Verification items for the finished model (mm, model axes). A direction names the side the tool comes from. Coordinates: 2 decimals unless noted, no trailing zeros. Order: outer loops, then holes, each group sorted by start corner. A loop starts at its lowest first (then second) coordinate and runs counter-clockwise, first axis right, second up. Notation, with made-up numbers: (19, -29) -> (77, -29) arc R26 ccw to (77, -7) -> close; hole circle Ø2 at (66, 65.5). An arc over 180 degrees is marked (long way). Write item = value, one per line. Start each with the question number.
1. Thickness scan on line 1 along Z through (x, y) = (76.9, 8.5); line 2 along X through (y, z) = (4.5, -28); line 3 along X through (y, z) = (2, 5). Record the ranges inside material, lowest first. Write a range as from..to.
2. Cross-section at A-A on y = 4.75. Record the cut outline in (x, z), plus the area to 3 significant figures.
3. Release check for a two-part mould opening along Z. For faces 4 (the flat face through (9, 2, -5)), 5 (the conical face through (77.115, 2.379, -28.028)), 6 (the flat face through (12, 10, -27)) record: +Z half, -Z half, draft (parallel to the pull), parting line (faces both ways), or undercut.
4. Cross-section at C-C on x = 57.5. Record the cut outline in (y, z).
5. Go/stop test with flat-tipped pins: P1, Ø5, axis at x = 60, y = 1.5, coming from the +Z side; P2, Ø2, axis at y = 1, z = 4.5, coming from the +X side; P3, Ø2, axis at x = 11, z = 18, coming from the -Y side; P4, Ø4.5, axis at y = 1.5, z = -20.5, coming from the -X side. Record where each tip stops, or that it passes through.
6. Cross-section at B-B on z = 3.5. Record the cut outline in (x, y).
7. Set-up check for faces 1 (the flat face through (78, 10, 19)), 2 (the cylindrical face through (75.846, 6.451, -27.328)), 3 (the flat face through (13, 2, 6)): record each of +Z, -Z, +X, -X, +Y, -Y from which the full face is reachable in a straight line by a thin tool's end or side.
Autodesk Fusion 360 part; units mm, degrees
sketch "Schizzo9" plane through (0, 0, 0) normal (0, 1, 0) x (1, 0, 0)
  line L0 (11, 28) -> (76.9, 28)
  line L1 (76.9, 28) -> (76.9, -18)
  line L2 (76.9, -18) -> (11, -18)
  line L3 (11, -18) -> (11, 28)
  circle A0 centre (11, 28) radius 2.75
  circle A1 centre (76.9, 28) radius 2.75
  circle A2 centre (11, -18) radius 2.75
  circle A3 centre (76.9, -18) radius 2.75
  line L4 (11, 28) -> (9, 28)
  line L5 (11, 28) -> (13, 28)
  line L6 (9, 28) -> (9, -18)
  line L7 (13, 28) -> (13, -18)
  line L8 (76.9, 28) -> (74.9, 28)
  line L9 (76.9, 28) -> (78.9, 28)
  line L10 (78.9, 28) -> (78.9, -18)
  line L11 (74.9, 28) -> (74.9, -18)
  line L12 (78.9, 5) -> (78.9, 7)
  line L13 (78.9, 5) -> (78.9, 3)
  line L14 (78.9, 7) -> (9, 7)
  line L15 (78.9, 3) -> (9, 3)
  dimension "d99" = 65.9
  dimension "d100" = 46
  dimension "d101" = 5.5
  dimension "d102" = 5.5
  dimension "d103" = 5.5
  dimension "d104" = 5.5
  dimension "d105" = 2
  dimension "d106" = 2
  dimension "d107" = 2
  dimension "d108" = 2
  dimension "d109" = 2
  dimension "d110" = 2
extrude "Estrusione16" add sketch "Schizzo9" along normal blind 4 contours L3 A0 L7 L14 | L3 A0 L6 L14 | L3 L7 L14 L15 | L3 L6 L14 L15 | L7 L11 L14 L15 | L3 A2 L7 L15 | L3 A2 L6 L15 | L1 A1 L11 L14 | L1 L11 L14 L15 | L1 A1 L10 L14 | L1 A3 L11 L15 | L1 L10 L12 L13 L14 L15 | L1 A3 L10 L15
extrude "Estrusione17" add sketch "Schizzo9" along normal blind 10 contours L0 A0 L4 L5 L6 | L0 L3 A0 L5 L7 | L3 A0 L4 L6 | L0 A0 L7 | L0 A1 L8 L9 L10 | L0 A1 L11 | L0 L1 A1 L8 L11 | L2 L3 A2 L7 | L2 L3 A2 | L1 A1 L9 L10 | L2 A2 L7 | L2 A3 L11 | L1 L2 A3 L11 | L1 L2 A3
hole "Foratura9" at (11, 10, -28) direction (0, -1, 0) diameter 2.5 depth 7 tip angle 118
hole "Foratura10" at (76.9, 10, -28) direction (0, -1, 0) diameter 2.5 depth 7 tip angle 118
hole "Foratura11" at (76.9, 10, 18) direction (0, -1, 0) diameter 2.5 depth 7 tip angle 118
hole "Foratura12" at (11, 10, 18) direction (0, -1, 0) diameter 2.5 depth 7 tip angle 118
Worked out:
q1.line_1 = -30.75..-29.25, -26.75..-25.25, 15.25..16.75, 19.25..20.75
q1.line_2 = 8.25..9.75, 12.25..13.75, 74.15..75.65, 78.15..79.65
q1.line_3 = 9..13, 74.9..78.9
q2.outline = circle Ø5.5 at (11, -28); circle Ø5.5 at (11, 18); circle Ø5.5 at (76.9, -28); circle Ø5.5 at (76.9, 18); hole circle Ø2.5 at (11, -28); hole circle Ø2.5 at (11, 18); hole circle Ø2.5 at (76.9, -28); hole circle Ø2.5 at (76.9, 18)
q2.area = 75.4 mm²
q3.face_4 = undercut
q3.face_5 = undercut
q3.face_6 = draft
q4.outline = (0, -7) -> (4, -7) -> (4, -3) -> (0, -3) -> close
q5.P1 = -3
q5.P2 = 78.9
q5.P3 = 0
q5.P4 = 9
q6.outline = (9, 0) -> (13, 0) -> (13, 4) -> (9, 4) -> close; (74.9, 0) -> (78.9, 0) -> (78.9, 4) -> (74.9, 4) -> close
q7.face_1 = +Z, -Z, +X, -X, +Y
q7.face_2 = +Y
q7.face_3 = +Y, -Y
